```python
from build123d import *

# Parameters (mm, degrees)
F1_DEPTH = 25


with BuildPart() as f1:
    # F0 (on Top) → F1 (new body)
    with BuildSketch(Plane.XY):
        with BuildLine():
            Line((-64.169525, 22.113068), (-64.169525, -47.886932))
            Line((-64.169525, -47.886932), (-34.169525, -47.886932))
            Line((-34.169525, -47.886932), (-34.169525, -27.886932))
            ThreePointArc((-34.169525, -27.886932), (-24.169525, -17.886932), (-14.169525, -27.886932))
            Line((-14.169525, -27.886932), (-14.169525, -47.886932))
            Line((-14.169525, -47.886932), (45.830475, -47.886932))
            Line((45.830475, -47.886932), (45.830475, -27.886932))
            ThreePointArc((45.830475, -27.886932), (55.28729, -14.635985), (64.744104, -27.886932))
            Line((64.744104, -27.886932), (64.744104, -48.687104))
            Line((64.744104, -48.687104), (104.744104, -48.687104))
            Line((104.744104, -48.687104), (104.744104, -4.687104))
            Line((104.744104, -4.687104), (59.47641, 37.893837))
            Line((59.47641, 37.893837), (24.47641, 37.893837))
            Line((24.47641, 37.893837), (24.47641, 7.893837))
            ThreePointArc((24.47641, 7.893837), (9.144929, -6.407142), (-5.50748, 8.588831))
            Line((-5.50748, 8.588831), (-5.50748, 38.588831))
            Line((-5.50748, 38.588831), (-55.50748, 38.588831))
            ThreePointArc((-55.50748, 38.588831), (-61.872055, 31.420078), (-64.169525, 22.113068))
        make_face()
    extrude(amount=F1_DEPTH)


solid = f1.part
```
Geometry check sheet. Reference: the model listing, model coordinates, mm. A direction names the side the tool comes from. Give positions to 0.01 mm unless a question says otherwise; leave off trailing zeros. Write each loop counter-clockwise with the first axis right and the second up, starting at its lowest first coordinate (ties: lowest second). Pieces come first, ordered by that corner, then holes.
1) Release check for a two-part mould opening along Y. For faces 6 (the flat face through (45.83, -38, 12)), 7 (the cylindrical face through (55.02, -14.64, 12.32)), 8 (the flat face through (84, -48.687, 12)) record: pulls with the +Y half, pulls with the -Y half, needs draft (parallel to the pull), parting line crosses it, or undercut.
2) Section check C-C, the plane z = 5.75. Record the boundary of the cut face in (x, y), and give its area (3 significant figures).
3) Access from +Z, -Z, +X, -X, +Y, -Y to the whole of each face (thin tool, end or side, straight path). Record for faces 1 (the flat face through (24.476, 23, 12)), 2 (the flat face through (42, 37.894, 12)), 3 (the flat face through (-49, -47.887, 12)), 4 (the cylindrical face through (-61.81, 31.54, 12.32)), 5 (the flat face through (-34.17, -38, 12)).
4) Section check D-D, the plane x = 34.5. Record the boundary of the cut face in (y, z).
5) Section check B-B, the plane y = 20. Record the boundary of the cut face in (x, z), and give its area (3 significant figures).
6) Gauge pin test, flat ends, axial feed: pin 1 (8 mm diameter, centred on y = 8.5, z = 14, fed in from +X); pin 2 (2 mm diameter, centred on x = -3.5, y = -33.5, fed in from -Z); pin 3 (12.5 mm diameter, centred on x = 41.5, z = 13, fed in from +Y); pin 4 (5 mm diameter, centred on y = 2.5, z = 18, fed in from +X). Record the tip position at first contact, or that the pin passes through.
7) Section check A-A, the plane y = -40. Record the boundary of the cut face in (x, z), and give its area (3 significant figures).
8) Material ranges on L1, parallel to X at y = -34.5, z = 15.25; L2, parallel to Y at x = 55.5, z = 6.75; L3, parallel to X at y = -5, z = 18, recorded low to high.
Computed:
1. face 6: needs draft
1. face 7: undercut
1. face 8: pulls with the -Y half
2. outline: (-64.17, -47.89) - (-34.17, -47.89) - (-34.17, -27.89) arc R10 cw to (-14.17, -27.89) - (-14.17, -47.89) - (45.83, -47.89) - (45.83, -27.89) arc R10 cw (long way) to (64.74, -27.89) - (64.74, -48.69) - (104.74, -48.69) - (104.74, -4.69) - (59.48, 37.89) - (24.48, 37.89) - (24.48, 7.89) arc R15 cw to (-5.51, 8.59) - (-5.51, 38.59) - (-55.51, 38.59) arc R20 ccw to (-64.17, 22.11) - close
2. area: 11,200 mm2
3. face 1: +Z, -Z, +Y
3. face 2: +Z, -Z, +X, +Y
3. face 3: +Z, -Z, -X, -Y
3. face 4: +Z, -Z, -X, +Y
3. face 5: +Z, -Z, -Y
4. outline: (-47.89, 0) - (37.89, 0) - (37.89, 25) - (-47.89, 25) - close
5. outline: (-64.17, 0) - (-5.51, 0) - (-5.51, 25) - (-64.17, 25) - close; (24.48, 0) - (78.5, 0) - (78.5, 25) - (24.48, 25) - close
5. area: 2,820 mm2
6. pin 1: stops at x = 94.98
6. pin 2: stops at z = 0
6. pin 3: stops at y = 37.89
6. pin 4: stops at x = 99.76
7. outline: (-64.17, 0) - (-34.17, 0) - (-34.17, 25) - (-64.17, 25) - close; (-14.17, 0) - (45.83, 0) - (45.83, 25) - (-14.17, 25) - close; (64.74, 0) - (104.74, 0) - (104.74, 25) - (64.74, 25) - close
7. area: 3,250 mm2
8. L1: x = -64.17 to -34.17, -14.17 to 45.83, 64.74 to 104.74
8. L2: y = -14.64 to 37.89
8. L3: x = -64.17 to 3.14, 15.84 to 104.74
